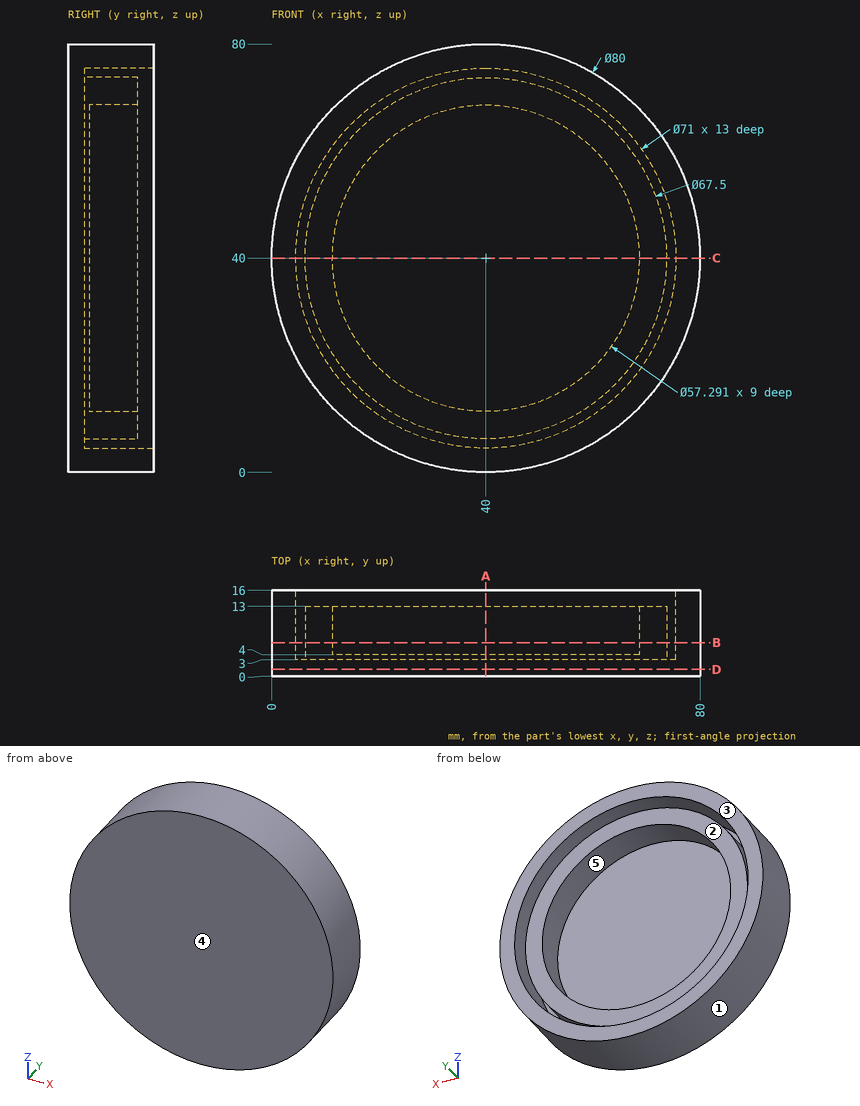
Geometry check sheet. Reference: drawing and pictorial views, mm from the part's lowest x, y, z. A direction names the side the tool comes from. Round coordinates to 2 decimals unless told otherwise and drop trailing zeros. Loops run counter-clockwise (first coordinate to the right, second up) from the corner with the lowest first, then second, coordinate; pieces in that order, holes last. Notation, with made-up numbers: (71, 87) -> (106, 87) arc R22 cw to (106, 112) -> close; hole circle Ø9 at (-15, -4). An arc over 180 degrees is marked (long way). Answer as a JSON object with one key per item and string values.
Q1. Go/stop test with flat-tipped pins: P1, Ø8, axis at x = 65, y = 3.5, coming from the +Z side; P2, Ø1, axis at y = 3.5, z = 51, coming from the -X side; P3, Ø1, axis at y = 2.5, z = 25, coming from the -X side. Record where each tip stops, or that it passes through.
Data:
{"P1": "stops at z = 74.04", "P2": "stops at x = 1.4", "P3": "stops at x = 2.72"}
Q2. Scan lines: line 1 (X direction, y = 10, z = 40); line 2 (Z direction, x = 34, y = 5); line 3 (Y direction, x = 46.5, z = 57.5). Record each from-to range of solid material in increasing order. Write a range as from..to.
Data:
{"line 1": "x = 0..4.5, 6.25..11.35, 68.65..73.75, 75.5..80", "line 2": "z = 0.45..5.01, 6.79..11.99, 68.01..73.21, 74.99..79.55", "line 3": "y = 0..4"}
Q3. Access from +Z, -Z, +X, -X, +Y, -Y to the whole of each face (thin tool, end or side, straight path). Record for the marked faces 4 and 5.
Data:
{"face 4": "+Z, -Z, +X, -X, -Y", "face 5": "+Y"}
Q4. Draft check along X on the marked faces 1, 2 and 3. Enter one of: pulls with the +X half, pulls with the -X half, needs draft (parallel to the pull), parting line crosses it, or undercut.
Data:
{"face 1": "parting line crosses it", "face 2": "undercut", "face 3": "needs draft"}
Q5. Section check A-A (x = 40). Record the boundary of the cut face in (y, z).
Data:
{"outline": "(0, 0) -> (16, 0) -> (16, 4.5) -> (3, 4.5) -> (3, 6.25) -> (13, 6.25) -> (13, 11.35) -> (4, 11.35) -> (4, 68.65) -> (13, 68.65) -> (13, 73.75) -> (3, 73.75) -> (3, 75.5) -> (16, 75.5) -> (16, 80) -> (0, 80) -> close"}
Q6. Section check D-D (y = 1.25). Record the boundary of the cut face in (x, z).
Data:
{"outline": "circle Ø80 at (40, 40)"}
Q7. Section check C-C (z = 40). Record the boundary of the cut face in (x, y).
Data:
{"outline": "(0, 0) -> (80, 0) -> (80, 16) -> (75.5, 16) -> (75.5, 3) -> (73.75, 3) -> (73.75, 13) -> (68.65, 13) -> (68.65, 4) -> (11.35, 4) -> (11.35, 13) -> (6.25, 13) -> (6.25, 3) -> (4.5, 3) -> (4.5, 16) -> (0, 16) -> close"}
Q8. Section check B-B (y = 6.25). Record the boundary of the cut face in (x, z).
Data:
{"outline": "circle Ø80 at (40, 40); circle Ø67.5 at (40, 40); hole circle Ø71 at (40, 40); hole circle Ø57.29 at (40, 40)"}
